```python
from build123d import *

# Parameters (mm, degrees)
SKETCH1_R           = 101.6
SKETCH1_R_2         = 3
BOSS_EXTRUDE1_DEPTH = 12.7
SKETCH7_R           = 101.6
SKETCH7_R_2         = 3
BOSS_EXTRUDE3_DEPTH = 6.35
SKETCH8_R           = 12.7
CUT_EXTRUDE1_DEPTH  = 6.35
CUT_EXTRUDE2_START  = -6.35
SKETCH9_R           = 12.7
CUT_EXTRUDE2_DEPTH  = 6.35
SKETCH10_R          = 101.6
CUT_EXTRUDE3_DEPTH  = 6.35
BOSS_EXTRUDE4_START = 3.175
SKETCH12_R          = 12.7
BOSS_EXTRUDE4_DEPTH = 3.175
SKETCH13_R          = 3
CUT_EXTRUDE6_DEPTH  = 3.175


with BuildPart() as part:
    # Sketch1 → Boss-Extrude1 (new body)
    with BuildSketch(Plane(origin=(0, 0, 0), x_dir=(1, 0, 0), z_dir=(0, 1, 0))):
        with Locations(Location((0, 0, 0), (0, 0, 270))):
            Circle(SKETCH1_R)
        with Locations(Location((0, 0, 0), (0, 0, 270))):
            Circle(SKETCH1_R_2, mode=Mode.SUBTRACT)
    extrude(amount=BOSS_EXTRUDE1_DEPTH)

    # Sketch7 → Boss-Extrude3 (add)
    with BuildSketch(Plane(origin=(0, 12.7, 0), x_dir=(1, 0, 0), z_dir=(0, 1, 0))):
        with Locations(Location((0, 0, 0), (0, 0, 270))):
            Circle(SKETCH7_R)
        with Locations(Location((0, 0, 0), (0, 0, 270))):
            Circle(SKETCH7_R_2, mode=Mode.SUBTRACT)
    extrude(amount=BOSS_EXTRUDE3_DEPTH)

    # Sketch8 → Cut-Extrude1 (cut)
    with BuildSketch(Plane(origin=(0, 19.05, 0), x_dir=(1, 0, 0), z_dir=(0, 1, 0))):
        with Locations(Location((0, 0, 0), (0, 0, 270))):
            Circle(SKETCH8_R)
    extrude(amount=-CUT_EXTRUDE1_DEPTH, mode=Mode.SUBTRACT)

    # Sketch9 → Cut-Extrude2 (cut)
    with BuildSketch(Plane.XZ.offset(CUT_EXTRUDE2_START)):
        with Locations(Location((0, 0, 0), (0, 0, 90))):
            Circle(SKETCH9_R)
    extrude(amount=CUT_EXTRUDE2_DEPTH, mode=Mode.SUBTRACT)

    # Sketch10 → Cut-Extrude3 (cut)
    with BuildSketch(Plane.XZ):
        with Locations(Location((0, 0, 0), (0, 0, 270))):
            Circle(SKETCH10_R)
    extrude(amount=-CUT_EXTRUDE3_DEPTH, mode=Mode.SUBTRACT)

    # Sketch12 → Boss-Extrude4 (add)
    with BuildSketch(Plane(origin=(0, 12.7, 0), x_dir=(1, 0, 0), z_dir=(0, 1, 0)).offset(BOSS_EXTRUDE4_START)):
        with Locations(Location((0, 0, 0), (0, 0, 270))):
            Circle(SKETCH12_R)
    extrude(amount=-BOSS_EXTRUDE4_DEPTH)

    # Sketch13 → Cut-Extrude6 (cut)
    with BuildSketch(Plane.XZ.offset(-12.7)):
        with Locations(Location((0, 0, 0), (0, 0, 270))):
            Circle(SKETCH13_R)
    extrude(amount=-CUT_EXTRUDE6_DEPTH, mode=Mode.SUBTRACT)


solid = part.part
```
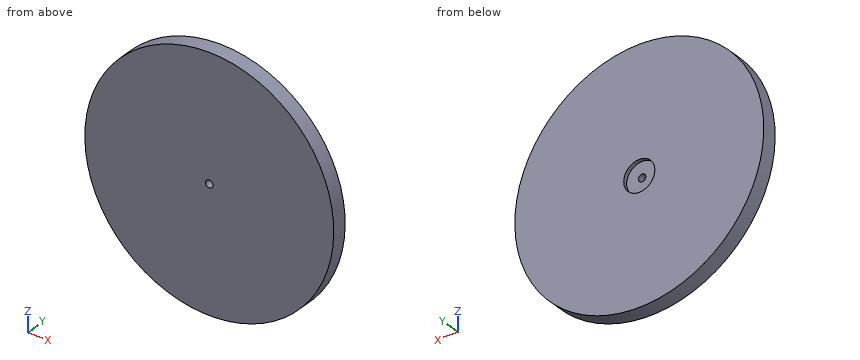
The model under review builds one solid part; all positions refer to its coordinate system, in mm. Round coordinates to 2 decimals unless told otherwise and drop trailing zeros. Write each loop counter-clockwise with the first axis right and the second up, starting at its lowest first coordinate (ties: lowest second). Pieces come first, ordered by that corner, then holes. Notation, with made-up numbers: M -7,41 L 3,41 A22 cw 3,52 Z; hole C 73,78.5 d9. An arc over 180 degrees is marked long. Use CSV: the item, a comma, the result in double quotes. Start each with the question number.
(1) We need section B-B, the plane x = 0. State the section outline as (y, z) points (3 decimals), then the cut area to 3 significant figures.
(2) We need section A-A, the plane z = 0. State the section outline as (x, y) points (3 decimals).
(3) We need section C-C, the plane x = -79. State the section outline as (y, z) points, then the cut area to 3 significant figures.
(4) We need section D-D, the plane z = -54. State the section outline as (x, y) points.
(5) Clearance check with flat-ended pins moving along their axes: P1, Ø1.5, axis at y = 8, z = 35.5, coming from the +X side; P2, Ø2, axis at x = 35, y = 14, coming from the +Z side; P3, Ø3, axis at x = -63, y = 17, coming from the +Z side. State where each tip first meets the part, or that it passes through.
(6) For line 1 along X through (y, z) = (17.5, 0); line 2 along X through (y, z) = (9.25, 0); line 3 along Z through (x, y) = (-6.5, 18.25), list the stretches that pass through material, from the lowest coordinate up.
Findings:
1,outline,"M 6.35,-101.6 L 19.05,-101.6 L 19.05,-12.7 L 15.875,-12.7 L 15.875,-3 L 6.35,-3 Z; M 6.35,3 L 15.875,3 L 15.875,12.7 L 19.05,12.7 L 19.05,101.6 L 6.35,101.6 Z"
1,area,"2,440 mm^2"
2,outline,"M -101.6,6.35 L -3,6.35 L -3,15.875 L -12.7,15.875 L -12.7,19.05 L -101.6,19.05 Z; M 3,6.35 L 101.6,6.35 L 101.6,19.05 L 12.7,19.05 L 12.7,15.875 L 3,15.875 Z"
3,outline,"M 6.35,-63.89 L 19.05,-63.89 L 19.05,63.89 L 6.35,63.89 Z"
3,area,"1,620 mm^2"
4,outline,"M -86.06,6.35 L 86.06,6.35 L 86.06,19.05 L -86.06,19.05 Z"
5,P1,"x = 95.47"
5,P2,"z = 95.74"
5,P3,"z = 80.87"
6,line 1,"-101.6 to -12.7, 12.7 to 101.6"
6,line 2,"-101.6 to -3, 3 to 101.6"
6,line 3,"-101.39 to -10.91, 10.91 to 101.39"
